Print and shaded views of the part. All mm, measured from the part's lowest x, y and z. A direction names the side the tool comes from. Coordinates: 2 decimals unless noted, no trailing zeros. Loops run counter-clockwise (first coordinate to the right, second up) from the corner with the lowest first, then second, coordinate; pieces in that order, holes last. Notation, with made-up numbers: M 30.25,-20.75 L 41.25,-20.75 A23 ccw 41.25,12.25 Z; hole C 70,60 d5. An arc over 180 degrees is marked long. Answer as a JSON object with one key per item and string values. Group by question number.
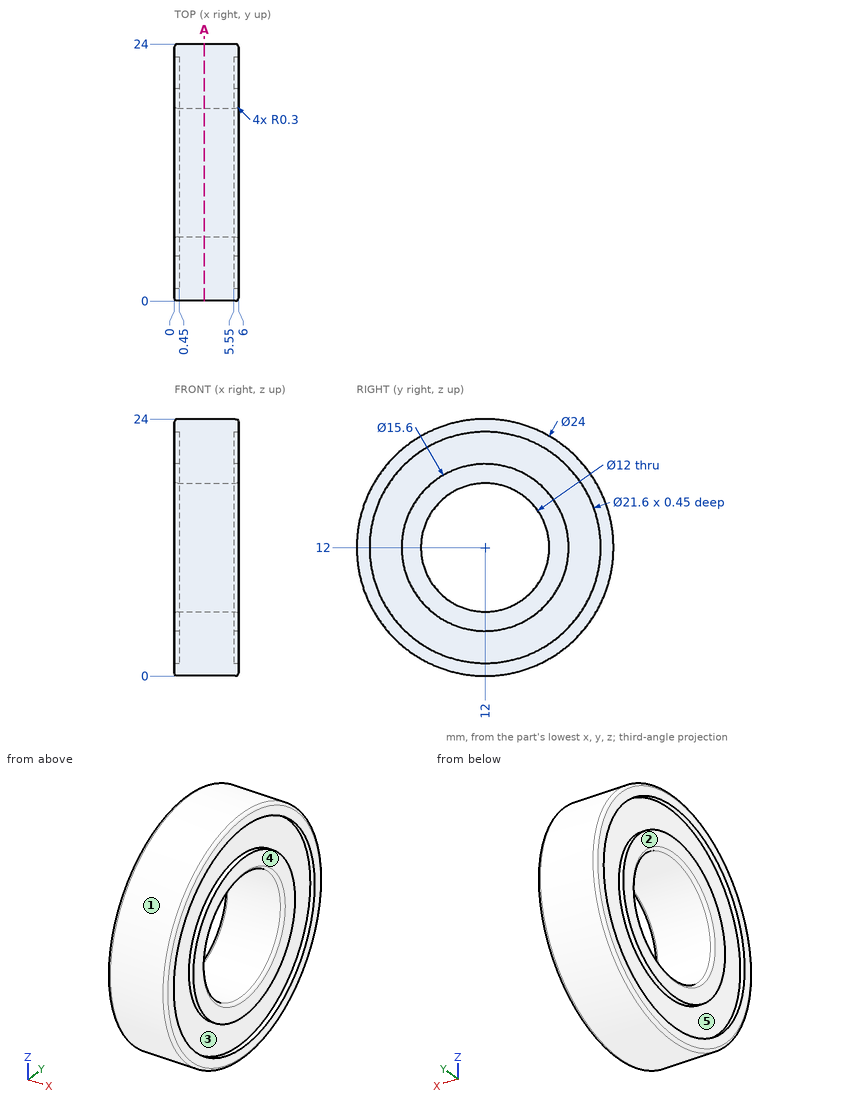
Item 1: Pin check, flat tips, straight feed: pin 1 (1.5 mm diameter, centred on y = 7, z = 3.5, fed in from +X); pin 2 (6.5 mm diameter, centred on y = 14, z = 13, fed in from +X). Stop position of each tip, or through.
Item 2: Pull direction Y, two halves, no side cores. Call the marked faces 1, 2 and 3: released by +Y, released by -Y, zero draft, split by the parting line, or undercut.
Item 3: Tool access for the marked faces 4 and 5: list every direction of +Z, -Z, +X, -X, +Y, -Y with a clear straight run to the whole face (end or side of a thin tool).
Item 4: Slice it at A-A, the plane x = 2.8. Write the cut outline in (y, z).
Item 5: Drill centre lines: L1, parallel to Z at x = 0.3, y = 12; L2, parallel to Y at x = 5.6, z = 18.5; L3, parallel to Z at x = 2.6, y = 12. Where is each one in solid material? Low to high. Write a range as from..to.
Computed:
{
 "1": {"pin 1": "x = 5.55", "pin 2": "through"},
 "2": {"face 1": "split by the parting line", "face 2": "zero draft", "face 3": "undercut"},
 "3": {"face 4": "+Z, -Z, +X, +Y, -Y", "face 5": "-X"},
 "4": {"outline": "C 12,12 d24; hole C 12,12 d12"},
 "5": {"L1": "0..1.2, 4.2..6, 18..19.8, 22.8..24", "L2": "1.91..3.38, 7.69..16.31, 20.62..22.09", "L3": "0..6, 18..24"}
}
